Part model, mm, in its own coordinate system. Face numbers are marked on the shaded views. A direction names the side the tool comes from. Give positions to 0.01 mm unless a question says otherwise; leave off trailing zeros. Order: outer loops, then holes, each group sorted by start corner. A loop starts at its lowest first (then second) coordinate and runs counter-clockwise, first axis right, second up. Notation, with made-up numbers: (13.25, -12) - (59.25, -12) arc R4 ccw to (59.25, -6) - close; hole circle Ø11 at (65.5, 64.25). An arc over 180 degrees is marked (long way). One line per item, written item: value.
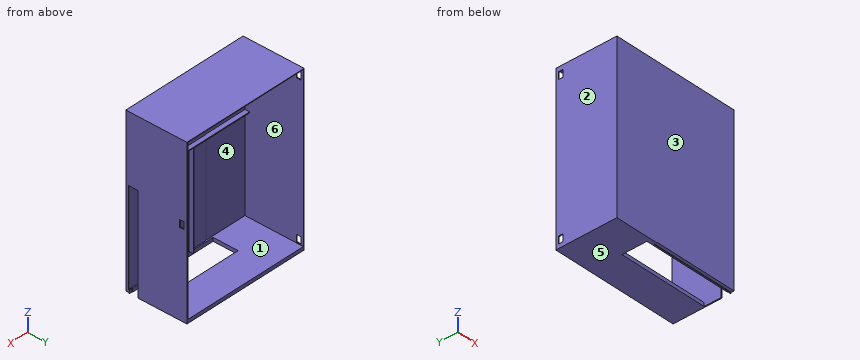
```python
from build123d import *

# Parameters (mm, degrees)
SKETCH1_W            = 76.15972441
SKETCH1_H            = 126.932874018
BOSS_EXTRUDE1_DEPTH  = 2.54
BOSS_EXTRUDE4_DEPTH  = 38.1
SHELL1_T             = -2.54
BOSS_EXTRUDE5_DEPTH  = 6.35
SKETCH16_W           = 76.15972441
SKETCH16_H           = 40.64
CUT_EXTRUDE7_DEPTH   = 7.112
SKETCH17_W           = 71.07972441
SKETCH17_H           = 3.09636258
CUT_EXTRUDE8_DEPTH   = 4.064
SKETCH19_W           = 35.651407884
SKETCH19_H           = 127.489236598
BOSS_EXTRUDE19_DEPTH = 2.286
SKETCH26_W           = 127.489236598
SKETCH26_H           = 38.354
CUT_EXTRUDE10_DEPTH  = 2.54
BOSS_EXTRUDE20_DEPTH = 40.64
SKETCH28_W           = 111.811132294
SKETCH28_H           = 15.936917459
BOSS_EXTRUDE21_DEPTH = 2.54
SKETCH34_W           = 111.811132294
SKETCH34_H           = 38.1
CUT_EXTRUDE12_DEPTH  = 5.08
BOSS_EXTRUDE23_DEPTH = 40.64
BOSS_EXTRUDE24_DEPTH = 6.35
BOSS_EXTRUDE28_DEPTH = 12.7
BOSS_EXTRUDE29_DEPTH = 27.94
SKETCH54_W           = 6.207163676
SKETCH54_H           = 3.981954056
CUT_EXTRUDE20_DEPTH  = 15.24
SKETCH55_W           = 6.104333468
SKETCH55_H           = 4.061705803
CUT_EXTRUDE21_DEPTH  = 15.24
SKETCH56_W           = 1.706619681
SKETCH56_H           = 138.67981609
CUT_EXTRUDE22_DEPTH  = 38.1
SKETCH57_W           = 5.678434708
SKETCH57_H           = 21.844
CUT_EXTRUDE23_DEPTH  = 38.1
CUT_EXTRUDE24_DEPTH  = 2.54
SKETCH59_W           = 110.26035724
SKETCH59_H           = 1.116448274
CUT_EXTRUDE25_DEPTH  = 38.1
SKETCH61_W           = 1.706619681
SKETCH61_H           = 14.640018444
CUT_EXTRUDE26_DEPTH  = 4.064
CUT_EXTRUDE28_DEPTH  = 0.762


with BuildPart() as part:
    # Sketch1 → Boss-Extrude1 (new body)
    with BuildSketch(Plane(origin=(0, 0, 0), x_dir=(1, 0, 0), z_dir=(0, 1, 0))):
        with Locations((0.933329956, -31.079887535)):
            Rectangle(SKETCH1_W, SKETCH1_H)
    extrude(amount=BOSS_EXTRUDE1_DEPTH)

    # Sketch7 → Boss-Extrude4 (add)
    with BuildSketch(Plane(origin=(0, 2.54, 0), x_dir=(1, 0, 0), z_dir=(0, 1, 0))):
        Polygon((-37.146532249, 32.386549474), (-37.146532249, -94.546324544), (39.013192161, -94.546324544), (39.013192161, 32.386549474), (39.013192161, 37.514912054), (-37.146532249, 37.514912054), align=None)
    extrude(amount=BOSS_EXTRUDE4_DEPTH)

    # Shell1
    shell1_openings = [part.faces().sort_by_distance(p)[0] for p in [
        (0.933329956, 40.64, 28.515706245),
    ]]
    offset(amount=SHELL1_T, openings=shell1_openings, kind=Kind.INTERSECTION)

    # Sketch12 → Boss-Extrude5 (add)
    with BuildSketch(Plane(origin=(0, 0, 0), x_dir=(1, 0, 0), z_dir=(0, 1, 0))):
        Polygon((-17.752421588, -53.993703886), (39.013192161, -53.993703886), (39.013192161, -53.328667969), (-17.752421588, -53.328667969), (-18.535651553, -53.328667969), (-18.344689589, 32.386549474), (-18.927981394, 32.386549474), (-18.927981394, -53.993703886), (-18.28148375, -53.993703886), align=None)
    extrude(amount=BOSS_EXTRUDE5_DEPTH)

    # Sketch16 → Cut-Extrude7 (cut)
    with BuildSketch(Plane(origin=(0, 0, -40.054912054), x_dir=(-1, 0, 0), z_dir=(0, 0, -1))):
        with Locations((-0.933329956, 20.32)):
            Rectangle(SKETCH16_W, SKETCH16_H)
    extrude(amount=-CUT_EXTRUDE7_DEPTH, mode=Mode.SUBTRACT)

    # Sketch17 → Cut-Extrude8 (cut)
    with BuildSketch(Plane(origin=(0, 7.62, 0), x_dir=(1, 0, 0), z_dir=(0, 1, 0))):
        with Locations((0.933329956, 31.394730764)):
            Rectangle(SKETCH17_W, SKETCH17_H)
    extrude(amount=-CUT_EXTRUDE8_DEPTH, mode=Mode.SUBTRACT)

    # Sketch19 → Boss-Extrude19 (add)
    with BuildSketch(Plane(origin=(0, 0, 0), x_dir=(1, 0, 0), z_dir=(0, 1, 0))):
        with Locations((-54.972236191, -30.801706245)):
            Rectangle(SKETCH19_W, SKETCH19_H)
    extrude(amount=BOSS_EXTRUDE19_DEPTH)

    # Sketch26 → Cut-Extrude10 (cut)
    with BuildSketch(Plane.ZY.offset(37.146532249)):
        with Locations((30.801706245, 21.463)):
            Rectangle(SKETCH26_W, SKETCH26_H)
    extrude(amount=-CUT_EXTRUDE10_DEPTH, mode=Mode.SUBTRACT)

    # Sketch27 → Boss-Extrude20 (add)
    with BuildSketch(Plane(origin=(0, 0, 0), x_dir=(1, 0, 0), z_dir=(0, 1, 0))):
        Polygon((-34.606532249, -94.546324544), (-72.797940133, -94.546324544), (-72.797940133, 32.942912054), (-34.606532249, 32.942912054), (-34.606532249, 29.846549474), (-72.080545398, 29.846549474), (-72.080545398, -92.006324544), (-70.104362866, -92.006324544), (-34.606532249, -92.006324544), align=None)
    extrude(amount=BOSS_EXTRUDE20_DEPTH)

    # Sketch28 → Boss-Extrude21 (add)
    with BuildSketch(Plane(origin=(0, 0, 0), x_dir=(1, 0, 0), z_dir=(0, 1, 0))):
        with Locations((-16.892373986, -102.514783274)):
            Rectangle(SKETCH28_W, SKETCH28_H)
    extrude(amount=BOSS_EXTRUDE21_DEPTH)

    # Sketch34 → Cut-Extrude12 (cut)
    with BuildSketch(Plane.XY.offset(97.086324544)):
        with Locations((-16.892373986, 21.59)):
            Rectangle(SKETCH34_W, SKETCH34_H)
    extrude(amount=-CUT_EXTRUDE12_DEPTH, mode=Mode.SUBTRACT)

    # Sketch36 → Boss-Extrude23 (add)
    with BuildSketch(Plane(origin=(0, 0, 0), x_dir=(1, 0, 0), z_dir=(0, 1, 0))):
        Polygon((-72.797940133, -92.006324544), (-72.797940133, -110.483242003), (39.013192161, -110.483242003), (39.013192161, -92.006324544), (36.473192161, -92.006324544), (36.473192161, -108.833266616), (-72.080545398, -108.833266616), (-72.080545398, -92.006324544), align=None)
    extrude(amount=BOSS_EXTRUDE23_DEPTH)

    # Sketch39 → Boss-Extrude24 (add)
    with BuildSketch(Plane(origin=(0, 0, 0), x_dir=(1, 0, 0), z_dir=(0, 1, 0))):
        Polygon((-19.575673417, -53.993703886), (-72.080545398, -53.993703886), (-72.080545398, -53.1861939), (-19.575673417, -53.1861939), (-18.927981394, -53.1861939), (-18.927981394, -53.993703886), align=None)
    extrude(amount=BOSS_EXTRUDE24_DEPTH)

    # Sketch51 → Boss-Extrude28 (add)
    with BuildSketch(Plane(origin=(0, 40.64, 0), x_dir=(1, 0, 0), z_dir=(0, 1, 0))):
        Polygon((-34.606532249, 32.942912054), (-34.606532249, 29.846549474), (-72.080545398, 29.846549474), (-72.080545398, -108.833266616), (-72.080545398, -109.553098124), (-72.080545398, -109.94971489), (38.179811842, -109.94971489), (38.179811842, -109.553098124), (38.179811842, 32.942912054), (39.013192161, 32.942912054), (39.013192161, -110.483242003), (-72.797940133, -110.483242003), (-72.797940133, 32.942912054), align=None)
    extrude(amount=BOSS_EXTRUDE28_DEPTH)

    # Sketch52 → Boss-Extrude29 (add)
    with BuildSketch(Plane(origin=(0, 53.34, 0), x_dir=(1, 0, 0), z_dir=(0, 1, 0))):
        Polygon((38.179811842, 32.942912054), (38.179811842, 29.846549474), (-34.606532249, 29.846549474), (-39.725324066, 29.846549474), (-39.725324066, 32.942912054), (-34.606532249, 32.942912054), align=None)
    extrude(amount=-BOSS_EXTRUDE29_DEPTH)

    # Sketch54 → Cut-Extrude20 (cut)
    with BuildSketch(Plane.ZY.offset(72.797940133)):
        with Locations((103.598874165, 49.097770639)):
            Rectangle(SKETCH54_W, SKETCH54_H)
        with Locations((-26.170821026, 49.097770639)):
            Rectangle(SKETCH54_W, SKETCH54_H)
    extrude(amount=-CUT_EXTRUDE20_DEPTH, mode=Mode.SUBTRACT)

    # Sketch55 → Cut-Extrude21 (cut)
    with BuildSketch(Plane(origin=(41.553192161, 0, 0), x_dir=(0, 0, -1), z_dir=(1, 0, 0))):
        with Locations((-43.456564529, 48.820045114)):
            Rectangle(SKETCH55_W, SKETCH55_H)
    extrude(amount=-CUT_EXTRUDE21_DEPTH, mode=Mode.SUBTRACT)

    # Sketch56 → Cut-Extrude22 (cut)
    with BuildSketch(Plane(origin=(0, 40.64, 0), x_dir=(1, 0, 0), z_dir=(0, 1, 0))):
        with Locations((37.326502002, -39.493358571)):
            Rectangle(SKETCH56_W, SKETCH56_H)
    extrude(amount=-CUT_EXTRUDE22_DEPTH, mode=Mode.SUBTRACT)

    # Sketch57 → Cut-Extrude23 (cut)
    with BuildSketch(Plane(origin=(0, 0, -32.942912054), x_dir=(-1, 0, 0), z_dir=(0, 0, -1))):
        with Locations((37.445749603, 14.478)):
            Rectangle(SKETCH57_W, SKETCH57_H)
    extrude(amount=-CUT_EXTRUDE23_DEPTH, mode=Mode.SUBTRACT)

    # Sketch58 → Cut-Extrude24 (cut)
    with BuildSketch(Plane(origin=(39.013192161, 0, 0), x_dir=(0, 0, -1), z_dir=(1, 0, 0))):
        Polygon((-51.99249987, 3.220445107), (32.386549474, 3.220445107), (32.942912054, 3.220445107), (32.942912054, 3.900890214), (32.942912054, 10.759981556), (-51.99249987, 10.759981556), align=None)
    extrude(amount=-CUT_EXTRUDE24_DEPTH, mode=Mode.SUBTRACT)

    # Sketch59 → Cut-Extrude25 (cut)
    with BuildSketch(Plane(origin=(0, 40.64, 0), x_dir=(1, 0, 0), z_dir=(0, 1, 0))):
        with Locations((-16.950366778, -109.391490753)):
            Rectangle(SKETCH59_W, SKETCH59_H)
    extrude(amount=-CUT_EXTRUDE25_DEPTH, mode=Mode.SUBTRACT)

    # Sketch61 → Cut-Extrude26 (cut)
    with BuildSketch(Plane.XY.offset(-29.846549474)):
        with Locations((37.326502002, 18.079990778)):
            Rectangle(SKETCH61_W, SKETCH61_H)
    extrude(amount=-CUT_EXTRUDE26_DEPTH, mode=Mode.SUBTRACT)

    # Sketch62 → Cut-Extrude28 (cut)
    with BuildSketch(Plane(origin=(0, 3.220445107, 0), x_dir=(1, 0, 0), z_dir=(0, 1, 0))):
        Polygon((38.179811842, -51.99249987), (39.013192161, -51.99249987), (39.013192161, 29.899968422), (38.179811842, 29.846549474), align=None)
    extrude(amount=-CUT_EXTRUDE28_DEPTH, mode=Mode.SUBTRACT)


solid = part.part
```
1) Cut at D-D, the plane x = -57.5. Give the cut face in (y, z), then the cut area to 3 significant figures.
Outcome:
outline: (0, -32.94) - (53.34, -32.94) - (53.34, -29.85) - (2.29, -29.85) - (2.29, 53.19) - (6.35, 53.19) - (6.35, 53.99) - (2.29, 53.99) - (2.29, 92.01) - (2.54, 92.01) - (2.54, 109.95) - (53.34, 109.95) - (53.34, 110.48) - (0, 110.48) - close
area: 521 mm^2
2) Cut at B-B, the plane y = 38. Give the cut face in (x, z), then the cut area to 3 significant figures.
Outcome:
outline: (-72.8, -32.94) - (39.01, -32.94) - (39.01, 110.48) - (-72.8, 110.48) - close; hole (-72.08, -29.85) - (38.18, -29.85) - (38.18, 109.95) - (-72.08, 109.95) - close
area: 623 mm^2
3) Mould opens along Z. For the marked faces 3, 4, 5 and 6 say: released by +Z, released by -Z, zero draft, split by the parting line, or undercut.
Outcome:
face 3: zero draft
face 4: undercut
face 5: released by -Z
face 6: undercut
4) Pin check, flat tips, straight feed: pin 1 (5 mm diameter, centred on x = 14.5, z = 43, fed in from +Y); pin 2 (18.5 mm diameter, centred on x = -51, z = -6, fed in from +Y); pin 3 (12 mm diameter, centred on x = 11, z = 54, fed in from +Y). Stop position of each tip, or through.
Outcome:
pin 1: stops at y = 2.54
pin 2: stops at y = 2.29
pin 3: stops at y = 6.35
5) Which spindle directions (+Z, -Z, +X, -X, +Y, -Y) get a long thin tool onto all of the face, cutting with end or side? Do the marked faces 1 and 2. Say none if no direction does.
Outcome:
face 1: +Y
face 2: +Z, -Z, -X, +Y, -Y
6) Cut at C-C, the plane z = -9. Give the cut face in (x, y), then the cut area to 3 significant figures.
Outcome:
outline: (-72.8, 0) - (39.01, 0) - (39.01, 2.46) - (38.18, 2.46) - (38.18, 2.54) - (-18.4, 2.54) - (-18.4, 6.35) - (-18.93, 6.35) - (-18.93, 2.54) - (-34.61, 2.54) - (-34.61, 2.29) - (-72.08, 2.29) - (-72.08, 53.34) - (-72.8, 53.34) - close; (38.18, 10.76) - (39.01, 10.76) - (39.01, 53.34) - (38.18, 53.34) - close
area: 348 mm^2
7) Drill centre lines: line 1 along X through (y, z) = (19, 41.5); line 2 along Z through (x, y) = (-32, 4); line 3 along Z through (x, y) = (13.5, 45). Where is each one in solid material? Low to high. Write a range as from..to.
Outcome:
line 1: x = -72.8..-72.08, 38.18..39.01
line 2: z = 53.19..53.99, 109.95..110.48
line 3: z = -32.94..-29.85, 109.95..110.48
8) Cut at A-A, the plane x = 30.5. Give the cut face in (y, z).
Outcome:
outline: (0, -32.39) - (2.54, -32.39) - (2.54, -32.94) - (3.56, -32.94) - (3.56, -29.85) - (2.54, -29.85) - (2.54, 53.33) - (6.35, 53.33) - (6.35, 53.99) - (2.54, 53.99) - (2.54, 109.95) - (53.34, 109.95) - (53.34, 110.48) - (0, 110.48) - close; (25.4, -32.94) - (53.34, -32.94) - (53.34, -29.85) - (25.4, -29.85) - close
